from build123d import *

# Parameters (mm, degrees)
BOSS_EXTRUDE1_DEPTH      = 24
SKETCH2_R                = 1.75
CUT_EXTRUDE1_DEPTH       = 24
SKETCH3_W                = 4
SKETCH3_H                = 7
CUT_EXTRUDE2_DEPTH       = 6.5
CHAMFER1_SIZE            = 1
CUT_EXTRUDE4_REACH       = 39.447
CUT_EXTRUDE5_DEPTH       = 38.446629
CHAMFER3_SIZE            = 1
CUT_EXTRUDE10_DEPTH      = 13
CUT_EXTRUDE10_DEPTH_BACK = 13
SKETCH11_W               = 4
SKETCH11_H               = 10
BOSS_EXTRUDE3_DEPTH      = 2
CHAMFER4_SIZE            = 1
SKETCH12_R               = 0.75
CUT_EXTRUDE6_DEPTH       = 2
CUT_EXTRUDE6_DEPTH_BACK  = 15
BOSS_EXTRUDE6_DEPTH      = 2
CHAMFER6_SIZE            = 1
CUT_EXTRUDE11_REACH      = 34.628
SKETCH19_R               = 0.75
SKETCH20_R               = 0.75
CUT_EXTRUDE12_DEPTH      = 1


with BuildPart() as part:
    # Sketch1 → Boss-Extrude1 (new body)
    with BuildSketch(Plane.XY):
        with BuildLine():
            Line((-3.25, 0), (-3.25, -28))
            Line((-3.25, -28), (3.25, -28))
            Line((3.25, -28), (3.25, 0))
            ThreePointArc((3.25, 0), (0, 3.25), (-3.25, 0))
        make_face()
    extrude(amount=BOSS_EXTRUDE1_DEPTH)

    # Sketch2 → Cut-Extrude1 (cut)
    with BuildSketch(Plane(origin=(0, 0, 0), x_dir=(-1, 0, 0), z_dir=(0, 0, -1))):
        Circle(SKETCH2_R)
    extrude(amount=-CUT_EXTRUDE1_DEPTH, mode=Mode.SUBTRACT)

    # Sketch3 → Cut-Extrude2 (cut)
    with BuildSketch(Plane.ZY.offset(3.25)):
        with Locations((5, 0.5)):
            Rectangle(SKETCH3_W, SKETCH3_H)
        with Locations((19, 0.5)):
            Rectangle(SKETCH3_W, SKETCH3_H)
        with Locations((12, 0.5)):
            Rectangle(SKETCH3_W, SKETCH3_H)
    extrude(amount=-CUT_EXTRUDE2_DEPTH, mode=Mode.SUBTRACT)

    # Chamfer1
    chamfer1_edges = [part.edges().sort_by_distance(p)[0] for p in [
        (3.25, -3, 5),
        (-3.25, -3, 5),
        (3.25, -3, 19),
        (-3.25, -3, 19),
        (3.25, -3, 12),
        (-3.25, -3, 12),
    ]]
    chamfer(chamfer1_edges, length=CHAMFER1_SIZE)

    # Sketch7 → Cut-Extrude4 (cut, up to next)
    with BuildSketch(Plane.ZY.offset(3.25), mode=Mode.PRIVATE) as cut_extrude4_sk1:
        Polygon((24, -28), (0, -4), (0, -28), align=None)
    cut_extrude4_tool1 = extrude(cut_extrude4_sk1.sketch, amount=-CUT_EXTRUDE4_REACH, mode=Mode.PRIVATE) & part.part
    add(cut_extrude4_tool1.solids().sort_by_distance((-3.25, -20, 8))[0], mode=Mode.SUBTRACT)

    # Sketch10 → Cut-Extrude5 (cut, through all)
    with BuildSketch(Plane(origin=(3.25, 0, 0), x_dir=(0, 0, -1), z_dir=(1, 0, 0))):
        Polygon((-24, -14), (-17, -21), (-24, -28), align=None)
    extrude(amount=-CUT_EXTRUDE5_DEPTH, mode=Mode.SUBTRACT)

    # Chamfer3
    chamfer3_edges = [part.edges().sort_by_distance(p)[0] for p in [
        (-3.25, -7, 24),
        (3.25, -2, 0),
        (3.25, -7, 24),
        (3.25, -17.5, 20.5),
        (-3.25, -17.5, 20.5),
        (-3.25, -2, 0),
        (0, 3.25, 0),
        (0, 3.25, 24),
    ]]
    chamfer(chamfer3_edges, length=CHAMFER3_SIZE)

    # Sketch18 → Cut-Extrude10 (cut, two sides)
    with BuildSketch(Plane(origin=(11.810029, -8.350951, 8.350951), x_dir=(-0.4082482904638629, 0.2886751345948129, 0.8660254037844388), z_dir=(-0.7071067811865475, 0.5000000000000001, -0.4999999999999999))) as cut_extrude10_sk:
        with BuildLine():
            ThreePointArc((6.229669, -8.809395), (6.383996, -10.861584), (8.267375, -11.691148))
            Line((8.267375, -11.691148), (9.17169, -11.339876))
            ThreePointArc((9.17169, -11.339876), (9.793137, -10.626285), (10.016989, -9.706883))
            ThreePointArc((10.016989, -9.706883), (8.936391, -7.930735), (6.862289, -8.07389))
            Line((6.862289, -8.07389), (6.229669, -8.809395))
        make_face()
        with BuildLine():
            Line((2.829335, -12.762736), (3.406685, -13.579233))
            Line((3.406685, -13.579233), (8.267375, -11.691148))
            ThreePointArc((8.267375, -11.691148), (6.383996, -10.861584), (6.229669, -8.809395))
            Line((6.229669, -8.809395), (2.829335, -12.762736))
        make_face()
    extrude(amount=CUT_EXTRUDE10_DEPTH, mode=Mode.SUBTRACT)
    extrude(cut_extrude10_sk.sketch, amount=-CUT_EXTRUDE10_DEPTH_BACK, mode=Mode.SUBTRACT)

    # Sketch11 → Boss-Extrude3 (add)
    with BuildSketch(Plane.ZY.offset(3.25)):
        with Locations((12, -9)):
            Rectangle(SKETCH11_W, SKETCH11_H)
    extrude(amount=BOSS_EXTRUDE3_DEPTH)

    # Chamfer4
    chamfer4_edges = [part.edges().sort_by_distance(p)[0] for p in [
        (-5.25, -9, 10),
        (-5.25, -14, 12),
        (-5.25, -9, 14),
        (-5.25, -4, 12),
    ]]
    chamfer(chamfer4_edges, length=CHAMFER4_SIZE)

    # Sketch12 → Cut-Extrude6 (cut, two sides)
    with BuildSketch(Plane(origin=(0, -4, 0), x_dir=(1, 0, 0), z_dir=(0, 1, 0))) as cut_extrude6_sk:
        with Locations(Location((-3.75, -12, 0), (0, 0, 48.189685))):
            Circle(SKETCH12_R)
    extrude(amount=CUT_EXTRUDE6_DEPTH, mode=Mode.SUBTRACT)
    extrude(cut_extrude6_sk.sketch, amount=-CUT_EXTRUDE6_DEPTH_BACK, mode=Mode.SUBTRACT)

    # Sketch14 → Boss-Extrude6 (add)
    with BuildSketch(Plane(origin=(3.25, 0, 0), x_dir=(0, 0, -1), z_dir=(1, 0, 0))):
        Polygon((-14, -4), (-7, -11), (-4, -8), (-8, -4), align=None)
    extrude(amount=BOSS_EXTRUDE6_DEPTH)

    # Chamfer6
    chamfer6_edges = [part.edges().sort_by_distance(p)[0] for p in [
        (5.25, -4, 11),
        (5.25, -9.5, 5.5),
        (5.25, -6, 6),
        (5.25, -7.5, 10.5),
    ]]
    chamfer(chamfer6_edges, length=CHAMFER6_SIZE)

    # Cut-Extrude11: up to this plane
    cut_extrude11_end = Plane(origin=(5.25, -4, 0), z_dir=(0, 1, 0))
    # Sketch19 → Cut-Extrude11 (cut, up to the surface)
    with BuildSketch(Plane(origin=(0, -2, -2), x_dir=(1, 0, 0), z_dir=(0, -0.7071067811865475, -0.7071067811865476)), mode=Mode.PRIVATE) as cut_extrude11_sk1:
        with Locations(Location((3.75, 10.606602, 0), (0, 0, 311.810315))):
            Circle(SKETCH19_R)
    cut_extrude11_tool1 = split(extrude(cut_extrude11_sk1.sketch, amount=-CUT_EXTRUDE11_REACH, mode=Mode.PRIVATE), bisect_by=cut_extrude11_end, keep=Keep.BOTH, mode=Mode.PRIVATE)
    add(cut_extrude11_tool1.solids().sort_by_distance((3.75, -9.5, 5.5))[0], mode=Mode.SUBTRACT)

    # Sketch20 → Cut-Extrude12 (cut)
    with BuildSketch(Plane(origin=(0, -4, 0), x_dir=(1, 0, 0), z_dir=(0, 1, 0))):
        with Locations((3.75, -11)):
            Circle(SKETCH20_R)
    extrude(amount=CUT_EXTRUDE12_DEPTH, mode=Mode.SUBTRACT)


solid = part.part
The model under review builds one solid part; all positions refer to its coordinate system, in mm. A direction names the side the tool comes from. Round coordinates to 2 decimals unless told otherwise and drop trailing zeros. Order: outer loops, then holes, each group sorted by start corner. A loop starts at its lowest first (then second) coordinate and runs counter-clockwise, first axis right, second up. Notation, with made-up numbers: (63.5, -30) -> (70.5, -30) arc R26 cw to (70.5, -3) -> close; hole circle Ø2 at (1, 49.25). An arc over 180 degrees is marked (long way). Write item = value, one per line. Start each with the question number.
Item 1: Consider section B-B on y = -1. Count the separate pieces of the cut face and the enclosed holes in it, plus the area to 3 significant figures.
Item 2: Consider section A-A on x = -3.75. Write out the cut boundary in (y, z), plus the area to 3 significant figures.
Item 3: For line 1 along Z through (x, y) = (-2.25, -1); line 2 along X through (y, z) = (-7.75, 12); line 3 along Z through (x, y) = (-3.75, -6.75), list the stretches that pass through material, from the lowest coordinate up.
Item 4: For faces 1 (the face through (4, -4, 13)), 2 (the face through (-4, -14, 13)), 3 (the face through (2.76, -3.51, 11.97)), 4 (the face through (-2.74, -3.49, 4.97)), list the 3-axis set-ups (+Z, -Z, +X, -X, +Y, -Y) from which the entire face can be reached by the end or side of a thin tool; tool diameter is ignored.
Item 5: Clearance check with flat-ended pins moving along their axes: pin 1 Ø4 at (x, z) = (-1.5, 5) entering from -Y; pin 2 Ø1.1 at (x, z) = (-3.5, 13.5) entering from -Y; pin 3 Ø2 at (x, y) = (2.5, -7) entering from -Z; pin 4 Ø3 at (x, y) = (0, 0) entering from +Z. State where each tip first meets the part, or that it passes through.
Item 6: Mouldability with a two-part tool opening along Z and no side actions: class faces 5 (the face through (-1.617, -0.67, 15.479)), 6 (the face through (-4.496, -8.607, 12.074)), 7 (the face through (-2.76, -2.47, 0.51)), 8 (the face through (2.76, -3.51, 4.97)) as released by +Z, released by -Z, zero draft, split by the parting line, or undercut.
Conclusion:
q1.separate_pieces = 8
q1.enclosed_holes = 0
q1.area = 41.5 mm2
q2.outline = (-14, 10) -> (-4, 10) -> (-4, 11.25) -> (-14, 11.25) -> close; (-14, 12.75) -> (-4, 12.75) -> (-4, 14) -> (-14, 14) -> close
q2.area = 25.0 mm2
q3.line_1 = 0 to 3, 7 to 10, 14 to 17, 21 to 24
q3.line_2 = -5.25 to -4.5, -3 to 3.25
q3.line_3 = 10 to 11.25, 12.75 to 14
q4.face_1 = +Z, -Z, +X, +Y
q4.face_2 = +Z, -Z, -X, -Y
q4.face_3 = +X, +Y
q4.face_4 = -X, +Y
q5.pin_1 = -11
q5.pin_2 = -17.99
q5.pin_3 = 2
q5.pin_4 = through
q6.face_5 = zero draft
q6.face_6 = undercut
q6.face_7 = released by -Z
q6.face_8 = undercut
